from build123d import *

# Parameters (mm, degrees)
SKETCH1_R           = 8.75
BOSS_EXTRUDE1_DEPTH = 55
SKETCH2_R           = 10
BOSS_EXTRUDE2_DEPTH = 27
BOSS_EXTRUDE3_START = 12
SKETCH3_R           = 10
BOSS_EXTRUDE3_DEPTH = 12
SKETCH4_R           = 4.5
BOSS_EXTRUDE4_DEPTH = 8
CUT_EXTRUDE1_START  = -121.5
CUT_EXTRUDE1_DEPTH  = 121.5
CUT_EXTRUDE2_START  = -17.5
CUT_EXTRUDE2_DEPTH  = 17.5
SKETCH7_R           = 2.5
CUT_EXTRUDE3_DEPTH  = 85.545845551
SKETCH8_R           = 2.5
CUT_EXTRUDE4_DEPTH  = 56.5
CUT_EXTRUDE5_START  = -133.5
CUT_EXTRUDE5_DEPTH  = 133.5
SKETCH10_R          = 1.5
CUT_EXTRUDE6_DEPTH  = 2
SKETCH11_R          = 1.5
CUT_EXTRUDE7_DEPTH  = 2
BOSS_EXTRUDE5_DEPTH = 14
BOSS_EXTRUDE6_DEPTH = 14


with BuildPart() as part:
    # Sketch1 → Boss-Extrude1 (new body)
    with BuildSketch(Plane.XY):
        Circle(SKETCH1_R)
    extrude(amount=BOSS_EXTRUDE1_DEPTH)

    # Sketch2 → Boss-Extrude2 (add)
    with BuildSketch(Plane.XY.offset(55)):
        Circle(SKETCH2_R)
    extrude(amount=BOSS_EXTRUDE2_DEPTH)

    # Sketch3 → Boss-Extrude3 (add)
    with BuildSketch(Plane(origin=(0, 0, 0), x_dir=(-1, 0, 0), z_dir=(0, 0, -1)).offset(BOSS_EXTRUDE3_START)):
        with Locations(Location((0, 0, 0), (0, 0, 180))):
            Circle(SKETCH3_R)
    extrude(amount=-BOSS_EXTRUDE3_DEPTH)

    # Sketch4 → Boss-Extrude4 (add)
    with BuildSketch(Plane(origin=(0, 0, -12), x_dir=(-1, 0, 0), z_dir=(0, 0, -1))):
        Circle(SKETCH4_R)
    extrude(amount=BOSS_EXTRUDE4_DEPTH)

    # Sketch5 → Cut-Extrude1 (cut)
    with BuildSketch(Plane.XY.offset(82).offset(CUT_EXTRUDE1_START)):
        with BuildLine():
            Line((-9, 4.358898944), (-9, -4.358898944))
            ThreePointArc((-9, -4.358898944), (-10, 0), (-9, 4.358898944))
        make_face()
        with BuildLine():
            Line((9, 4.358898944), (9, -4.358898944))
            ThreePointArc((9, -4.358898944), (10, 0), (9, 4.358898944))
        make_face()
    extrude(amount=CUT_EXTRUDE1_DEPTH, mode=Mode.SUBTRACT)

    # Sketch6 → Cut-Extrude2 (cut)
    with BuildSketch(Plane.XY.offset(82).offset(CUT_EXTRUDE2_START)):
        with BuildLine():
            Line((-3.211619504, 9.470242878), (-2.786893563, -9.603813007))
            ThreePointArc((-2.786893563, -9.603813007), (0.210299095, -9.99778847), (3.188273823, -9.478127981))
            Line((3.188273823, -9.478127981), (2.810550168, 9.596916575))
            ThreePointArc((2.810550168, 9.596916575), (-0.210299095, 9.99778847), (-3.211619504, 9.470242878))
        make_face()
    extrude(amount=CUT_EXTRUDE2_DEPTH, mode=Mode.SUBTRACT)

    # Sketch7 → Cut-Extrude3 (cut, through all)
    with BuildSketch(Plane(origin=(9, 0, 0), x_dir=(0, 0, -1), z_dir=(1, 0, 0))):
        with Locations((-74, 0)):
            Circle(SKETCH7_R)
    extrude(amount=-CUT_EXTRUDE3_DEPTH, mode=Mode.SUBTRACT)

    # Sketch8 → Cut-Extrude4 (cut)
    with BuildSketch(Plane(origin=(0, 0, -20), x_dir=(-1, 0, 0), z_dir=(0, 0, -1))):
        Circle(SKETCH8_R)
    extrude(amount=-CUT_EXTRUDE4_DEPTH, mode=Mode.SUBTRACT)

    # Sketch9 → Cut-Extrude5 (cut)
    with BuildSketch(Plane.XY.offset(82).offset(CUT_EXTRUDE5_START)):
        with BuildLine():
            Line((-4.358898944, 9), (4.358898944, 9))
            ThreePointArc((4.358898944, 9), (3.597127672, 9.330630874), (2.810550168, 9.596916575))
            ThreePointArc((2.810550168, 9.596916575), (-0.210299095, 9.99778847), (-3.211619504, 9.470242878))
            ThreePointArc((-3.211619504, 9.470242878), (-3.79255448, 9.252920108), (-4.358898944, 9))
        make_face()
        with BuildLine():
            Line((-4.358898944, -9), (4.358898944, -9))
            ThreePointArc((4.358898944, -9), (3.781151383, -9.257585766), (3.188273823, -9.478127981))
            ThreePointArc((3.188273823, -9.478127981), (0.210299095, -9.99778847), (-2.786893563, -9.603813007))
            ThreePointArc((-2.786893563, -9.603813007), (-3.585628979, -9.335055695), (-4.358898944, -9))
        make_face()
    extrude(amount=CUT_EXTRUDE5_DEPTH, mode=Mode.SUBTRACT)

    # Sketch10 → Cut-Extrude6 (cut)
    with BuildSketch(Plane(origin=(0, 9, 0), x_dir=(1, 0, 0), z_dir=(0, 1, 0))):
        with Locations(Location((0, 5, 0), (0, 0, 180))):
            Circle(SKETCH10_R)
    extrude(amount=-CUT_EXTRUDE6_DEPTH, mode=Mode.SUBTRACT)

    # Sketch11 → Cut-Extrude7 (cut)
    with BuildSketch(Plane(origin=(0, 9, 0), x_dir=(1, 0, 0), z_dir=(0, 1, 0))):
        with Locations(Location((0, -59.5, 0), (0, 0, 180))):
            Circle(SKETCH11_R)
    extrude(amount=-CUT_EXTRUDE7_DEPTH, mode=Mode.SUBTRACT)

    # Sketch13 → Boss-Extrude5 (add)
    with BuildSketch(Plane(origin=(0, 9, 0), x_dir=(1, 0, 0), z_dir=(0, 1, 0))):
        Polygon((4.993693542, 2.102352999), (5.006282685, 7.875841965), (0.012589143, 10.773488967), (-4.993693542, 7.897647001), (-5.006282685, 2.124158035), (-0.012589143, -0.773488967), align=None)
    extrude(amount=BOSS_EXTRUDE5_DEPTH)

    # Sketch14 → Boss-Extrude6 (add)
    with BuildSketch(Plane(origin=(0, 9, 0), x_dir=(1, 0, 0), z_dir=(0, 1, 0))):
        Polygon((1.10432569, -65.166903749), (5.459845453, -61.377077773), (4.355519763, -55.710174024), (-1.10432569, -53.833096251), (-5.459845453, -57.622922227), (-4.355519763, -63.289825976), align=None)
    extrude(amount=BOSS_EXTRUDE6_DEPTH)


solid = part.part
The model under review builds one solid part; all positions refer to its coordinate system, in mm. A direction names the side the tool comes from. Round coordinates to 2 decimals unless told otherwise and drop trailing zeros. Order: outer loops, then holes, each group sorted by start corner. A loop starts at its lowest first (then second) coordinate and runs counter-clockwise, first axis right, second up. Notation, with made-up numbers: (41.25, -4.75) -> (75.25, -4.75) arc R6 ccw to (75.25, -0.75) -> close; hole circle Ø10 at (-23, -21). An arc over 180 degrees is marked (long way). Use CSV: the item, a comma, the result in double quotes. Start each with the question number.
(1) Insertion check: pin 1 (5 mm diameter, centred on x = -0.5, z = 30.5, fed in from -Y); pin 2 (8 mm diameter, centred on x = 5.5, z = 32, fed in from -Y); pin 3 (1.2 mm diameter, centred on x = 2.5, z = 76.5, fed in from +Y); pin 4 (5 mm diameter, centred on y = 12.5, z = 10, fed in from -X). Each pin has a flat end and moves straight along its axis. Give the tip position at first contact, or say it passes through.
(2) Wall thickness on probe 1 along Z at (x, y) = (0, 8.1); probe 2 along Y at (x, z) = (0, 6); probe 3 along Y at (x, z) = (0, -1): over which ranges is each line inside the solid? List them lowest first. Write a range as from..to.
(3) Consider section A-A on y = 14.5. Write out the cut boundary in (x, z), and give its area (3 significant figures).
(4) Mouldability with a two-part tool opening along Y and no side actions: class faces 1 (the face through (0, 7, 60)), 2 (the face through (0, 0, 64.5)), 3 (the face through (-7.1, -7.04, 68.31)), 4 (the face through (3.5, 9, -0.5)) as pulls with the +Y half, pulls with the -Y half, needs draft (parallel to the pull), parting line crosses it, or undercut.
(5) Consider section C-C on x = -6.5. Write out the cut boundary in (y, z).
(6) Consider section D-D on y = 0. State how many separate pieces and enclosed holes the cut face has, and give its area (3 significant figures).
(7) Consider section B-B on z = 75. Write out the cut boundary in (x, y), and give its area (3 significant figures).
(8) Tool access review of faces 5 (the face through (-4, 9, 70)), 6 (the face through (0, 0, 36.5)), 7 (the face through (2.456, 15.902, -0.644)): name each direction out of +Z, -Z, +X, -X, +Y, -Y from which nothing blocks a thin tool from reaching the whole face with its end or side.
Responses:
1,pin 1,"y = -8.75"
1,pin 2,"y = -8.62"
1,pin 3,"y = 9"
1,pin 4,"through"
2,probe 1,"-12..-6.5, -3.5..58, 61..64.5"
2,probe 2,"-8.75..-2.5, 2.5..8.75"
2,probe 3,"-9..-2.5, 2.5..23"
3,outline,"(-5.46, 57.62) -> (-1.1, 53.83) -> (4.36, 55.71) -> (5.46, 61.38) -> (1.1, 65.17) -> (-4.36, 63.29) -> close; (-5.01, -2.12) -> (-4.99, -7.9) -> (0.01, -10.77) -> (5.01, -7.88) -> (4.99, -2.1) -> (-0.01, 0.77) -> close"
3,area,"173 mm²"
4,face 1,"undercut"
4,face 2,"needs draft"
4,face 3,"pulls with the -Y half"
4,face 4,"pulls with the +Y half"
5,outline,"(-7.6, -12) -> (7.6, -12) -> (7.6, 0) -> (5.86, 0) -> (5.86, 55) -> (7.6, 55) -> (7.6, 82) -> (-7.6, 82) -> (-7.6, 55) -> (-5.86, 55) -> (-5.86, 0) -> (-7.6, 0) -> close; hole circle Ø5 at (0, 74)"
6,separate pieces,"3"
6,enclosed holes,"0"
6,area,"1,290 mm²"
7,outline,"(-9, -4.36) arc R10 ccw to (-4.36, -9) -> (-2.8, -9) -> (-2.95, -2.29) -> (-9, -2.29) -> close; (-9, 2.29) -> (-3.05, 2.29) -> (-3.2, 9) -> (-4.36, 9) arc R10 ccw to (-9, 4.36) -> close; (2.82, 9) -> (2.96, 2.29) -> (9, 2.29) -> (9, 4.36) arc R10 ccw to (4.36, 9) -> close; (3.05, -2.29) -> (3.18, -9) -> (4.36, -9) arc R10 ccw to (9, -4.36) -> (9, -2.29) -> close"
7,area,"128 mm²"
8,face 5,"+Z, -X, +Y"
8,face 6,"-Z"
8,face 7,"+X, +Y"
